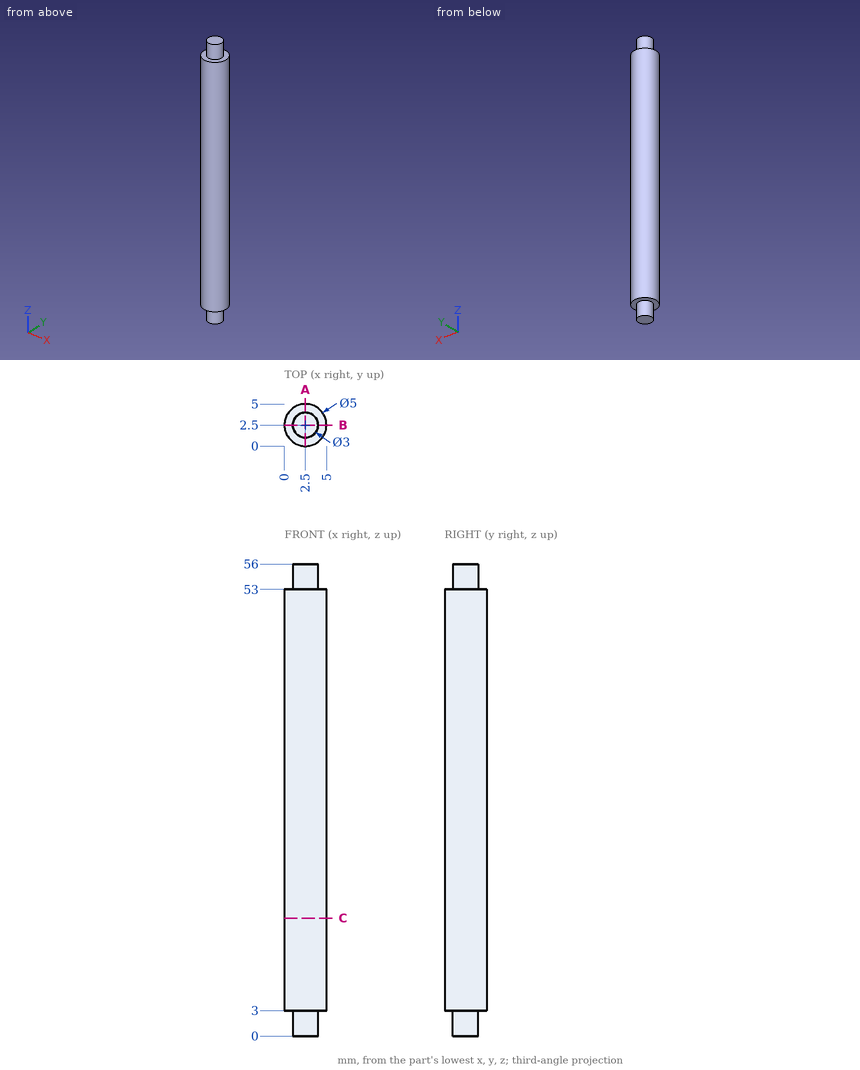
The drawing under review shows one solid part. Ordinate dimensions are in mm from its lowest x, y, z. Round coordinates to 2 decimals unless told otherwise and drop trailing zeros. Loops run counter-clockwise (first coordinate to the right, second up) from the corner with the lowest first, then second, coordinate; pieces in that order, holes last. Notation, with made-up numbers: (89, 39.5) - (112, 39.5) arc R20 cw to (112, 55.5) - close; hole circle Ø8 at (44.25, -23). An arc over 180 degrees is marked (long way). Use a Markdown table: item, result. Add a question column.
Q1. Add section C-C (z = 14). State the section outline as (x, y) points.
Q2. Add section A-A (x = 2.5). State the section outline as (y, z) points.
Q3. For probe 1 along Z at (x, y) = (4.2, 2.2); probe 2 along X at (y, z) = (3.95, 35); probe 3 along Y at (x, z) = (2.3, 30), list the stretches that pass through material, from the lowest coordinate up.
Worked answers:
| question | item | result |
|---|---|---|
| 1 | outline | circle Ø5 at (2.5, 2.5) |
| 2 | outline | (0, 3) - (1, 3) - (1, 0) - (4, 0) - (4, 3) - (5, 3) - (5, 53) - (4, 53) - (4, 56) - (1, 56) - (1, 53) - (0, 53) - close |
| 3 | probe 1 | 3 to 53 |
| 3 | probe 2 | 0.46 to 4.54 |
| 3 | probe 3 | 0.01 to 4.99 |
